CAD build for the part. Positions are in the model's coordinates, mm. A direction names the side the tool comes from. Round coordinates to 2 decimals unless told otherwise and drop trailing zeros. Write each loop counter-clockwise with the first axis right and the second up, starting at its lowest first coordinate (ties: lowest second). Pieces come first, ordered by that corner, then holes. Notation, with made-up numbers: (88, -23.75) - (121, -23.75) arc R19 cw to (121, -15.75) - close; hole circle Ø4 at (6, 6.5). An arc over 180 degrees is marked (long way). Answer in a Markdown table with one row per item.
```python
from build123d import *

# Parameters (mm, degrees)
BOSS_EXTRU_1_DEPTH           = 3
COQUE1_T                     = 1.5
ESQUISSE2_R                  = 2.5
ESQUISSE2_R_2                = 1.6
BOSS_EXTRU_2_DEPTH           = 1.4
ENL_V_MAT_EXTRU_1_DEPTH      = 30.925950277
ENL_V_MAT_EXTRU_1_DEPTH_BACK = 30.925950277
ESQUISSE3_R                  = 1.6


with BuildPart() as part:
    # Esquisse1 → Boss.-Extru.1 (new body)
    with BuildSketch(Plane.XY):
        with BuildLine():
            Line((-24.48, -10.5), (24.48, -10.5))
            ThreePointArc((24.48, -10.5), (25.378025612, -10.128025612), (25.75, -9.23))
            Line((25.75, -9.23), (25.75, 9.23))
            ThreePointArc((25.75, 9.23), (25.378025612, 10.128025612), (24.48, 10.5))
            Line((24.48, 10.5), (-24.48, 10.5))
            ThreePointArc((-24.48, 10.5), (-25.378025612, 10.128025612), (-25.75, 9.23))
            Line((-25.75, 9.23), (-25.75, -9.23))
            ThreePointArc((-25.75, -9.23), (-25.378025612, -10.128025612), (-24.48, -10.5))
        make_face()
    extrude(amount=BOSS_EXTRU_1_DEPTH)

    # Coque1
    coque1_openings = [part.faces().sort_by_distance(p)[0] for p in [
        (0, 0, 3),
    ]]
    offset(amount=COQUE1_T, openings=coque1_openings, kind=Kind.INTERSECTION)

    # Esquisse2 → Boss.-Extru.2 (add)
    # profile 1 of 4: a face of its own
    with BuildSketch(Plane.XY):
        with Locations((20.32, 5.08)):
            Circle(ESQUISSE2_R)
        with Locations((20.32, 5.08)):
            Circle(ESQUISSE2_R_2, mode=Mode.SUBTRACT)
    # profile 2 of 4: a face of its own
    with BuildSketch(Plane.XY):
        with Locations((-20.955, -5.08)):
            Circle(ESQUISSE2_R)
        with Locations((-20.955, -5.08)):
            Circle(ESQUISSE2_R_2, mode=Mode.SUBTRACT)
    # profile 3 of 4: a face of its own
    with BuildSketch(Plane.XY):
        with Locations((-20.955, 5.08)):
            Circle(ESQUISSE2_R)
        with Locations((-20.955, 5.08)):
            Circle(ESQUISSE2_R_2, mode=Mode.SUBTRACT)
    # profile 4 of 4: a face of its own
    with BuildSketch(Plane.XY):
        with Locations((20.32, -5.08)):
            Circle(ESQUISSE2_R)
        with Locations((20.32, -5.08)):
            Circle(ESQUISSE2_R_2, mode=Mode.SUBTRACT)
    extrude(amount=BOSS_EXTRU_2_DEPTH)

    # Esquisse3 → Enlèv. mat.-Extru.1 (cut, two sides: drawn at the far end of the back side and taken through both)
    with BuildSketch(Plane.XY.offset(-ENL_V_MAT_EXTRU_1_DEPTH_BACK)):
        with Locations((20.32, 5.08)):
            Circle(ESQUISSE3_R)
        with Locations((-20.955, 5.08)):
            Circle(ESQUISSE3_R)
        with Locations((-20.955, -5.08)):
            Circle(ESQUISSE3_R)
        with Locations((20.32, -5.08)):
            Circle(ESQUISSE3_R)
    extrude(amount=ENL_V_MAT_EXTRU_1_DEPTH + ENL_V_MAT_EXTRU_1_DEPTH_BACK, mode=Mode.SUBTRACT)


solid = part.part
```
Q1. Drill centre lines: line 1 (X direction, y = -5.08, z = -0.45) (3 decimals); line 2 (Y direction, x = 20.32, z = -0.9); line 3 (Y direction, x = 13, z = 1.75). Where is each one in solid material? Low to high.
Computed:
| item | result |
|---|---|
| line 1 | x = -27.25 to -22.555, -19.355 to 18.72, 21.92 to 27.25 |
| line 2 | y = -12 to -6.68, -3.48 to 3.48, 6.68 to 12 |
| line 3 | y = -12 to -10.5, 10.5 to 12 |
Q2. Saw through at B-B on y = 5.08. List the corners of the cut face in (x, z) (3 decimals).
Computed:
| item | result |
|---|---|
| outline | (-27.25, -1.5) - (-22.555, -1.5) - (-22.555, 1.4) - (-23.455, 1.4) - (-23.455, 0) - (-25.75, 0) - (-25.75, 3) - (-27.25, 3) - close; (-19.355, -1.5) - (18.72, -1.5) - (18.72, 1.4) - (17.82, 1.4) - (17.82, 0) - (-18.455, 0) - (-18.455, 1.4) - (-19.355, 1.4) - close; (21.92, -1.5) - (27.25, -1.5) - (27.25, 3) - (25.75, 3) - (25.75, 0) - (22.82, 0) - (22.82, 1.4) - (21.92, 1.4) - close |
Q3. Flat gauge pins, fed straight in: pin 1 (1 mm diameter, centred on x = 5, y = -4, fed in from +Z); pin 2 (2.5 mm diameter, centred on x = -20.5, y = -5.5, fed in from +Z). Where does each tip first touch, or does it go through?
Computed:
| item | result |
|---|---|
| pin 1 | stops at z = 0 |
| pin 2 | stops at z = 1.4 |
Q4. Saw through at C-C on z = 1.95. List the corners of the cut face in (x, y), then the cut area to 3 significant figures.
Computed:
| item | result |
|---|---|
| outline | (-27.25, -9.23) arc R2.77 ccw to (-24.48, -12) - (24.48, -12) arc R2.77 ccw to (27.25, -9.23) - (27.25, 9.23) arc R2.77 ccw to (24.48, 12) - (-24.48, 12) arc R2.77 ccw to (-27.25, 9.23) - close; hole (-25.75, -9.23) arc R1.27 ccw to (-24.48, -10.5) - (24.48, -10.5) arc R1.27 ccw to (25.75, -9.23) - (25.75, 9.23) arc R1.27 ccw to (24.48, 10.5) - (-24.48, 10.5) arc R1.27 ccw to (-25.75, 9.23) - close |
| area | 221 mm2 |
Q5. Saw through at A-A on x = 20.32. List the corners of the cut face in (y, z).
Computed:
| item | result |
|---|---|
| outline | (-12, -1.5) - (-6.68, -1.5) - (-6.68, 1.4) - (-7.58, 1.4) - (-7.58, 0) - (-10.5, 0) - (-10.5, 3) - (-12, 3) - close; (-3.48, -1.5) - (3.48, -1.5) - (3.48, 1.4) - (2.58, 1.4) - (2.58, 0) - (-2.58, 0) - (-2.58, 1.4) - (-3.48, 1.4) - close; (6.68, -1.5) - (12, -1.5) - (12, 3) - (10.5, 3) - (10.5, 0) - (7.58, 0) - (7.58, 1.4) - (6.68, 1.4) - close |
Q6. Pull direction Y, two halves, no side cores. Call faces 1 (the flat face through (0, 12, 1)), 2 (the cylindrical face through (-18.646, -6.038, 0.69)), 3 (the flat face through (0, 0, -1.5)): released by +Y, released by -Y, zero draft, split by the parting line, or undercut.
Computed:
| item | result |
|---|---|
| face 1 | released by +Y |
| face 2 | undercut |
| face 3 | zero draft |
Q7. Saw through at D-D on x = 10. List the corners of the cut face in (y, z).
Computed:
| item | result |
|---|---|
| outline | (-12, -1.5) - (12, -1.5) - (12, 3) - (10.5, 3) - (10.5, 0) - (-10.5, 0) - (-10.5, 3) - (-12, 3) - close |
Q8. 3-axis set-ups, long thin cutter, end or side, ignore diameter. For faces 4 (the cylindrical face through (-26.46, -11.167, 0.719)), 5 (the flat face through (20, 3, 1.4)): which of +Z, -Z, +X, -X, +Y, -Y reach the whole face in a straight line?
Computed:
| item | result |
|---|---|
| face 4 | +Z, -Z, -X, -Y |
| face 5 | +Z |
